```python
from build123d import *

# Parameters (mm, degrees)
F1_DEPTH    = 45
F2_T1_DEPTH = 45
F3_W        = 4.5
F3_H        = 8.5
F4_DEPTH    = 1.5


# Not quite as in the source:
# - a fillet or chamfer that OpenCascade refuses, or shapes differently, is made with other operations: its cross-section is extruded or revolved along the edge and cut away or added


with BuildPart() as f1:
    # F0 (on Top) → F1 (new body)
    with BuildSketch(Plane.XY):
        Polygon((36.5, 0), (0, 0), (-36.5, 0), (-36.5, 8), (-33.5, 8), (-33.5, 9.5), (-38, 9.5), (-38, -1.5), (-34.25, -1.5), (-32.75, -1.5), (0, -1.5), (32.75, -1.5), (34.25, -1.5), (38, -1.5), (38, 9.5), (33.5, 9.5), (33.5, 8), (36.5, 8), align=None)
        Polygon((-32.75, -1.5), (-34.25, -1.5), (-34.25, -11.5), (-28.25, -11.5), (-28.25, -10), (-32.75, -10), align=None)
        Polygon((34.25, -11.5), (34.25, -1.5), (32.75, -1.5), (32.75, -10), (28.25, -10), (28.25, -11.5), align=None)
    extrude(amount=F1_DEPTH)

    # F2: fillet of radius 6 on 2 edges, made by hand

    # F2_s2 → F2_t1 (join)
    with BuildSketch(Plane.XY):
        with BuildLine():
            ThreePointArc((-38, -1.5), (-35.2750628145, -3.7080468991), (-34.25, -7.0621488653))
            Line((-34.25, -7.0621488653), (-34.25, -1.5))
            Line((-34.25, -1.5), (-38, -1.5))
        make_face()
        with BuildLine():
            ThreePointArc((34.25, -7.0621488653), (35.2750628145, -3.7080468991), (38, -1.5))
            Line((38, -1.5), (34.25, -1.5))
            Line((34.25, -1.5), (34.25, -7.0621488653))
        make_face()
    extrude(amount=F2_T1_DEPTH)

    # F3 (on face) → F4 (join)
    with BuildSketch(Plane(origin=(0, 0, 0), x_dir=(1, 0, 0), z_dir=(0, 0, -1))):
        with BuildLine():
            Line((-38, -9.5), (-33.5, -9.5))
            Line((-33.5, -9.5), (-33.5, -8))
            Line((-33.5, -8), (-36.5, -8))
            Line((-36.5, -8), (-36.5, 0))
            Line((-36.5, 0), (-20, 0))
            Line((-20, 0), (20, 0))
            Line((20, 0), (36.5, 0))
            Line((36.5, 0), (36.5, -8))
            Line((36.5, -8), (33.5, -8))
            Line((33.5, -8), (33.5, -9.5))
            Line((33.5, -9.5), (38, -9.5))
            Line((38, -9.5), (38, 1.5))
            ThreePointArc((38, 1.5), (35.2750628145, 3.7080468991), (34.25, 7.0621488653))
            Line((34.25, 7.0621488653), (34.25, 11.5))
            Line((34.25, 11.5), (28.25, 11.5))
            Line((28.25, 11.5), (28.25, 10))
            Line((28.25, 10), (32.75, 10))
            Line((32.75, 10), (32.75, 1.5))
            Line((32.75, 1.5), (28.25, 1.5))
            Line((28.25, 1.5), (-28.25, 1.5))
            Line((-28.25, 1.5), (-32.75, 1.5))
            Line((-32.75, 1.5), (-32.75, 10))
            Line((-32.75, 10), (-28.25, 10))
            Line((-28.25, 10), (-28.25, 11.5))
            Line((-28.25, 11.5), (-34.25, 11.5))
            Line((-34.25, 11.5), (-34.25, 7.0621488653))
            ThreePointArc((-34.25, 7.0621488653), (-35.2750628145, 3.7080468991), (-38, 1.5))
            Line((-38, 1.5), (-38, -9.5))
        make_face()
        with Locations((-30.5, 5.75)):
            Rectangle(F3_W, F3_H)
        Polygon((-33.5, -8), (-33.5, -9.5), (-20, -9.5), (-20, 0), (-36.5, 0), (-36.5, -8), align=None)
        Polygon((36.5, 0), (20, 0), (20, -9.5), (33.5, -9.5), (33.5, -8), (36.5, -8), align=None)
        with Locations((30.5, 5.75)):
            Rectangle(F3_W, F3_H)
    extrude(amount=F4_DEPTH)


solid = f1.part
```
Model file for the job. Use its own axes, mm. A direction names the side the tool comes from. Coordinates: 2 decimals unless noted, no trailing zeros. Order: outer loops, then holes, each group sorted by start corner. A loop starts at its lowest first (then second) coordinate and runs counter-clockwise, first axis right, second up. Notation, with made-up numbers: (5.5, 1) -> (62.5, 1) arc R19 ccw to (62.5, 28) -> close; hole circle Ø2 at (-2, -8). An arc over 180 degrees is marked (long way). Answer as a JSON object with one key per item and string values. Group by question number.
1) Cut at A-A, the plane y = 4.5. Write the cut outline in (x, z), then the cut area to 3 significant figures.
2) Which spindle directions (+Z, -Z, +X, -X, +Y, -Y) get a long thin tool onto all of the face, cutting with end or side? Do faces 4 (the face through (-33.5, 9, 22)), 5 (the face through (-28.25, -11, 18)), 6 (the face through (36.5, 4, 22)), 7 (the face through (-34.25, -9, 22)). Say none if no direction does.
3) Cut at C-C, the plane x = 26. Write the cut outline in (y, z).
4) Pull direction X, two halves, no side cores. Call faces 1 (the face through (-1, 0, 22)), 2 (the face through (34.25, -9, 22)), 3 (the face through (-6, -1, 45)): +X half, -X half, draft (parallel to the pull), parting line (faces both ways), or undercut.
5) Cut at B-B, the plane z = 15.5. Write the cut outline in (x, y).
6) Cut at D-D, the plane y = -3.75. Write the cut outline in (x, z).
7) Flat gauge pins, fed straight in: pin 1 (23 mm diameter, centred on x = -4, z = 11, fed in from +Y); pin 2 (1.5 mm diameter, centred on x = 15, z = 37, fed in from -Y); pin 3 (3 mm diameter, centred on x = -26.5, y = 4, fed in from +Z). Where does each tip first touch, or does it go through?
8) Drill centre lines: L1, parallel to X at y = 6.25, z = 9; L2, parallel to X at y = -7.25, z = 3; L3, parallel to Y at x = 18, z = 14. Where is each one in solid material? Low to high.
Check values:
{
 "1": {"outline": "(-38, -1.5) -> (-20, -1.5) -> (-20, 0) -> (-36.5, 0) -> (-36.5, 45) -> (-38, 45) -> close; (20, -1.5) -> (38, -1.5) -> (38, 45) -> (36.5, 45) -> (36.5, 0) -> (20, 0) -> close", "area": "189 mm²"},
 "2": {"face 4": "+Z, +Y", "face 5": "+Z, -Z, -Y", "face 6": "+Z", "face 7": "+Z, -Z, -X, -Y"},
 "3": {"outline": "(-1.5, -1.5) -> (9.5, -1.5) -> (9.5, 0) -> (0, 0) -> (0, 45) -> (-1.5, 45) -> close"},
 "4": {"face 1": "undercut", "face 2": "+X half", "face 3": "draft"},
 "5": {"outline": "(-38, -1.5) arc R6 cw to (-34.25, -7.06) -> (-34.25, -11.5) -> (-28.25, -11.5) -> (-28.25, -10) -> (-32.75, -10) -> (-32.75, -1.5) -> (32.75, -1.5) -> (32.75, -10) -> (28.25, -10) -> (28.25, -11.5) -> (34.25, -11.5) -> (34.25, -7.06) arc R6 cw to (38, -1.5) -> (38, 9.5) -> (33.5, 9.5) -> (33.5, 8) -> (36.5, 8) -> (36.5, 0) -> (-36.5, 0) -> (-36.5, 8) -> (-33.5, 8) -> (-33.5, 9.5) -> (-38, 9.5) -> close"},
 "6": {"outline": "(-35.25, -1.5) -> (-28.25, -1.5) -> (-28.25, 0) -> (-32.75, 0) -> (-32.75, 45) -> (-35.25, 45) -> close; (28.25, -1.5) -> (35.25, -1.5) -> (35.25, 45) -> (32.75, 45) -> (32.75, 0) -> (28.25, 0) -> close"},
 "7": {"pin 1": "stops at y = 0", "pin 2": "stops at y = -1.5", "pin 3": "stops at z = 0"},
 "8": {"L1": "x = -38 to -36.5, 36.5 to 38", "L2": "x = -34.25 to -32.75, 32.75 to 34.25", "L3": "y = -1.5 to 0"}
}
